Build history of the part. All positions in model axes, mm. Face numbers are marked on the shaded views. A direction names the side the tool comes from. Coordinates: 2 decimals unless noted, no trailing zeros. Write each loop counter-clockwise with the first axis right and the second up, starting at its lowest first coordinate (ties: lowest second). Pieces come first, ordered by that corner, then holes.
```python
from build123d import *

# Parameters (mm, degrees)
F0_R      = 7.0358
F1_DEPTH  = 4.318
F2_SIZE2  = 4.2175894432
F2_SIZE   = 2.8448
F3_W      = 2.54
F3_H      = 2.5500503834
F4_DEPTH  = 8.128
F5_R      = 1.1351249509
F6_DEPTH  = 2.6416
F7_R      = 4.6971074758
F8_DEPTH  = 0.5588
F9_R      = 0.8130420693
F10_DEPTH = 12.446


with BuildPart() as f1:
    # F0 (on Top) → F1 (new body)
    with BuildSketch(Plane.XY):
        Circle(F0_R)
    extrude(amount=F1_DEPTH)

    # F2
    f2_edges = [f1.edges().sort_by_distance(p)[0] for p in [
        (-7.0358, 0, 4.318),
    ]]
    f2_side = f1.faces().sort_by_distance((0, 0, 4.318))[0]
    chamfer(f2_edges, length=F2_SIZE, length2=F2_SIZE2, reference=f2_side)

    # F3 (on Front) → F4 (join)
    with BuildSketch(Plane.XZ):
        with Locations((0, 1.7557573738)):
            Rectangle(F3_W, F3_H)
    extrude(amount=F4_DEPTH)

    # F5 (on face) → F6 (join)
    with BuildSketch(Plane.XZ.offset(8.128)):
        with Locations((0, 1.7557573738)):
            Circle(F5_R)
    extrude(amount=F6_DEPTH)

    # F7 (on face) → F8 (cut)
    with BuildSketch(Plane(origin=(0, 0, 0), x_dir=(1, 0, 0), z_dir=(0, 0, -1))):
        Circle(F7_R)
    extrude(amount=-F8_DEPTH, mode=Mode.SUBTRACT)

    # F9 (on face) → F10 (join)
    with BuildSketch(Plane.XZ.offset(10.7696)):
        with Locations((0, 1.7557573738)):
            Circle(F9_R)
    extrude(amount=F10_DEPTH)


solid = f1.part
```
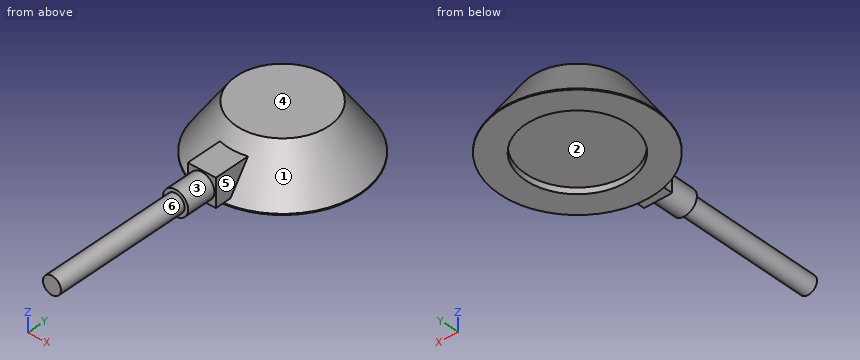
1. Saw through at B-B on y = 0. List the corners of the cut face in (x, z), plus the area to 3 significant figures.
Computed values:
outline: (-7.04, 0) - (-4.7, 0) - (-4.7, 0.56) - (4.7, 0.56) - (4.7, 0) - (7.04, 0) - (7.04, 0.1) - (4.19, 4.32) - (-4.19, 4.32) - (-7.04, 0.1) - close
area: 43.5 mm2
2. Saw through at A-A on x = 0. List the corners of the cut face in (y, z), plus the area to 3 significant figures.
Computed values:
outline: (-23.22, 0.94) - (-10.77, 0.94) - (-10.77, 0.62) - (-8.13, 0.62) - (-8.13, 0.48) - (-6.78, 0.48) - (-7.04, 0.1) - (-7.04, 0) - (-4.7, 0) - (-4.7, 0.56) - (4.7, 0.56) - (4.7, 0) - (7.04, 0) - (7.04, 0.1) - (4.19, 4.32) - (-4.19, 4.32) - (-5.06, 3.03) - (-8.13, 3.03) - (-8.13, 2.89) - (-10.77, 2.89) - (-10.77, 2.57) - (-23.22, 2.57) - close
area: 75.4 mm2
3. Saw through at D-D on y = -7.5. List the corners of the cut face in (x, z), plus the area to 3 significant figures.
Computed values:
outline: (-1.27, 0.48) - (1.27, 0.48) - (1.27, 3.03) - (-1.27, 3.03) - close
area: 6.48 mm2
4. Probe line 1 along Z through (x, y) = (-2.5, -1); line 2 along X through (y, z) = (-12, 1.8); line 3 along Y through (x, z) = (0, 0.45). List the from-to ranges inside material, lowest first.
Computed values:
line 1: z = 0.56 to 4.32
line 2: x = -0.81 to 0.81
line 3: y = -6.8 to -4.7, 4.7 to 6.8
5. Saw through at C-C on z = 2.25. List the corners of the cut face in (x, y), plus the area to 3 significant figures.
Computed values:
outline: (-1.27, -8.13) - (-1.02, -8.13) - (-1.02, -10.77) - (-0.65, -10.77) - (-0.65, -23.22) - (0.65, -23.22) - (0.65, -10.77) - (1.02, -10.77) - (1.02, -8.13) - (1.27, -8.13) - (1.27, -5.44) arc R5.59 ccw (long way) to (-1.27, -5.44) - close
area: 126 mm2
6. Mould opens along Y. For the marked faces 1, 2 and 3 say: +Y half, -Y half, draft (parallel to the pull), parting line (faces both ways), or undercut.
Computed values:
face 1: parting line
face 2: undercut
face 3: draft
7. Flat gauge pins, fed straight in: pin 1 (4 mm diameter, centred on x = -1.5, y = -20, fed in from -Z); pin 2 (2 mm diameter, centred on x = -0.5, y = -7, fed in from +Z); pin 3 (1.5 mm diameter, centred on x = 4, z = 3.5, fed in from -Y). Where does each tip first touch, or does it go through?
Computed values:
pin 1: stops at z = 0.94
pin 2: stops at z = 3.03
pin 3: stops at y = -3.74
8. 3-axis set-ups, long thin cutter, end or side, ignore diameter. For the marked faces 4, 5 and 6: which of +Z, -Z, +X, -X, +Y, -Y reach the whole face in a straight line?
Computed values:
face 4: +Z, +X, -X, +Y, -Y
face 5: +Z, +X, -Y
face 6: -Y
